Could you check a few things on this model? Use its own coordinates, in mm. Face numbers are marked on the shaded views. A direction names the side the tool comes from. Give positions to 0.01 mm unless a question says otherwise; leave off trailing zeros. Loops run counter-clockwise (first coordinate to the right, second up) from the corner with the lowest first, then second, coordinate; pieces in that order, holes last. Notation, with made-up numbers: (79.25, -35.5) - (88.25, -35.5) arc R17 ccw to (88.25, -22.5) - close; hole circle Ø3 at (26.5, 24.25). An arc over 180 degrees is marked (long way). One line per item, written item: value. Start each with the question number.
Q1. I'm going to push flat-ended pins straight in: P1, Ø1.5, axis at y = 16.5, z = 13, coming from the -X side; P2, Ø6, axis at y = 12, z = 14, coming from the +X side; P3, Ø7.5, axis at x = 7, y = 11.5, coming from the -Z side. Where does each tip first touch, or does it pass through?
Q2. I want a section at D-D (z = 7). Please give me the cut outline in (x, y).
Q3. If we mould it in two halves opening along X, with no side actions, what happens to the marked faces 1, 2, 3 and 4? For each: released by +X, released by -X, zero draft, split by the parting line, or undercut.
Q4. I want a section at A-A (y = 6). Please give me the cut outline in (x, z).
Q5. I want a section at C-C (y = 15.5). Please give me the cut outline in (x, z).
Q6. If I drill on line 1 (Y direction, x = 7, z = 15); line 2 (Z direction, x = 17, y = 1.4); line 3 (X direction, y = 15, z = 23.25), over which ranges is the centre line in solid material (lowest first)? Write a range as from..to.
Q7. For the marked faces 5, 6 and 7, which set-ups out of +Z, -Z, +X, -X, +Y, -Y let a thin tool reach every point of the face, with its end or its side?
Q8. I want a section at B-B (x = 17). Please give me the cut outline in (y, z), then the cut area to 3 significant figures.
```python
from build123d import *

# Parameters (mm, degrees)
CROQUIS1_W                 = 42
CROQUIS1_H                 = 5
SALIENTE_EXTRUIR1_DEPTH    = 30
CORTAR_EXTRUIR1_DEPTH      = 15
CORTAR_EXTRUIR1_DEPTH_BACK = 21
CROQUIS2_R                 = 1.6
CORTAR_EXTRUIR2_DEPTH      = 2.8
CROQUIS4_W                 = 7
CROQUIS4_H                 = 20
SALIENTE_EXTRUIR2_DEPTH    = 20
REDONDEO1_R                = 9
CORTAR_EXTRUIR3_DEPTH      = 11
CORTAR_EXTRUIR3_DEPTH_BACK = 23
CROQUIS5_R                 = 2


with BuildPart() as part:
    # Croquis1 → Saliente-Extruir1 (new body)
    with BuildSketch(Plane.XY):
        with Locations((0, 2.5)):
            Rectangle(CROQUIS1_W, CROQUIS1_H)
    extrude(amount=SALIENTE_EXTRUIR1_DEPTH)

    # Croquis2 → Cortar-Extruir1 (cut, two sides: drawn at the far end of the back side and taken through both)
    with BuildSketch(Plane(origin=(0, 5, 0), x_dir=(1, 0, 0), z_dir=(0, 1, 0)).offset(-CORTAR_EXTRUIR1_DEPTH_BACK)):
        with Locations((-17, -15)):
            Circle(CROQUIS2_R)
        with Locations((17, -15)):
            Circle(CROQUIS2_R)
    extrude(amount=CORTAR_EXTRUIR1_DEPTH + CORTAR_EXTRUIR1_DEPTH_BACK, mode=Mode.SUBTRACT)

    # Croquis3 → Cortar-Extruir2 (cut)
    with BuildSketch(Plane(origin=(0, 5, 0), x_dir=(1, 0, 0), z_dir=(0, 1, 0))):
        Polygon((15.383419246, -17.8), (13.766838493, -15), (15.383419246, -12.2), (18.616580754, -12.2), (20.233161507, -15), (18.616580754, -17.8), align=None)
        Polygon((-13.766838493, -15), (-15.383419246, -12.2), (-18.616580754, -12.2), (-20.233161507, -15), (-18.616580754, -17.8), (-15.383419246, -17.8), align=None)
    extrude(amount=-CORTAR_EXTRUIR2_DEPTH, mode=Mode.SUBTRACT)

    # Croquis4 → Saliente-Extruir2 (add)
    with BuildSketch(Plane(origin=(0, 5, 0), x_dir=(1, 0, 0), z_dir=(0, 1, 0))):
        with Locations((-7, -15)):
            Rectangle(CROQUIS4_W, CROQUIS4_H)
        with Locations((7, -15)):
            Rectangle(CROQUIS4_W, CROQUIS4_H)
    extrude(amount=SALIENTE_EXTRUIR2_DEPTH)

    # Redondeo1
    redondeo1_edges = [part.edges().sort_by_distance(p)[0] for p in [
        (7, 25, 5),
        (7, 25, 25),
        (-7, 25, 25),
        (-7, 25, 5),
    ]]
    fillet(redondeo1_edges, radius=REDONDEO1_R)

    # Croquis5 → Cortar-Extruir3 (cut, two sides: drawn at the far end of the back side and taken through both)
    with BuildSketch(Plane(origin=(10.5, 0, 0), x_dir=(0, 0, -1), z_dir=(1, 0, 0)).offset(-CORTAR_EXTRUIR3_DEPTH_BACK)):
        with Locations(Location((-15, 16, 0), (0, 0, 180))):
            Circle(CROQUIS5_R)
    extrude(amount=CORTAR_EXTRUIR3_DEPTH + CORTAR_EXTRUIR3_DEPTH_BACK, mode=Mode.SUBTRACT)


solid = part.part
```
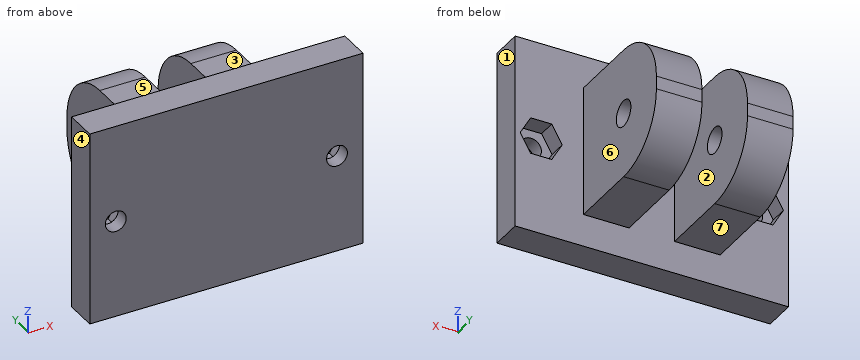
Worked answers:
1. P1: stops at x = -10.5
1. P2: stops at x = 10.5
1. P3: stops at z = 5
2. outline: (-21, 0) - (21, 0) - (21, 5) - (10.5, 5) - (10.5, 21.66) - (3.5, 21.66) - (3.5, 5) - (-3.5, 5) - (-3.5, 21.66) - (-10.5, 21.66) - (-10.5, 5) - (-21, 5) - close
3. face 1: released by +X
3. face 2: undercut
3. face 3: zero draft
3. face 4: released by -X
4. outline: (-10.5, 5) - (-3.5, 5) - (-3.5, 25) - (-10.5, 25) - close; (3.5, 5) - (10.5, 5) - (10.5, 25) - (3.5, 25) - close
5. outline: (-10.5, 5) - (-3.5, 5) - (-3.5, 13.06) - (-10.5, 13.06) - close; (-10.5, 16.94) - (-3.5, 16.94) - (-3.5, 25) - (-10.5, 25) - close; (3.5, 5) - (10.5, 5) - (10.5, 13.06) - (3.5, 13.06) - close; (3.5, 16.94) - (10.5, 16.94) - (10.5, 25) - (3.5, 25) - close
6. line 1: y = 0..14, 18..25
6. line 2: z = 0..13.4, 16.6..30
6. line 3: x = -10.5..-3.5, 3.5..10.5
7. face 5: +Z, +X, -X, +Y
7. face 6: +Z, -Z, +X, +Y
7. face 7: -Z, +X, -X, +Y
8. outline: (0, 0) - (5, 0) - (5, 12.2) - (2.2, 12.2) - (2.2, 13.4) - (0, 13.4) - close; (0, 16.6) - (2.2, 16.6) - (2.2, 17.8) - (5, 17.8) - (5, 30) - (0, 30) - close
8. area: 127 mm²
